```python
from build123d import *

# Parameters (mm, degrees)
SKETCH2_W           = 190.5
SKETCH2_H           = 203.2
BOSS_EXTRUDE1_DEPTH = 6
SKETCH5_R           = 2.5
CUT_EXTRUDE6_DEPTH  = 7
SKETCH6_W           = 31.9
SKETCH6_H           = 11
SKETCH6_R           = 2
CUT_EXTRUDE8_DEPTH  = 10


with BuildPart() as part:
    # Sketch2 → Boss-Extrude1 (new body)
    with BuildSketch(Plane(origin=(0, 0, 0), x_dir=(1, 0, 0), z_dir=(0, 1, 0))):
        Rectangle(SKETCH2_W, SKETCH2_H)
    extrude(amount=BOSS_EXTRUDE1_DEPTH)

    # Sketch5 → Cut-Extrude6 (cut, through all)
    with BuildSketch(Plane(origin=(0, 6, 0), x_dir=(1, 0, 0), z_dir=(0, 1, 0))):
        with Locations((-78.187036158, 94.165073798)):
            Circle(SKETCH5_R)
        with Locations((0, 94.165073798)):
            Circle(SKETCH5_R)
        with Locations((78.187036158, 0)):
            Circle(SKETCH5_R)
        with Locations((-78.187036158, 0)):
            Circle(SKETCH5_R)
        with Locations((78.187036158, 94.165073798)):
            Circle(SKETCH5_R)
        with Locations((-78.187036158, -94.165073798)):
            Circle(SKETCH5_R)
        with Locations((78.187036158, -94.165073798)):
            Circle(SKETCH5_R)
    extrude(amount=-CUT_EXTRUDE6_DEPTH, mode=Mode.SUBTRACT)

    # Sketch6 → Cut-Extrude8 (cut)
    with BuildSketch(Plane(origin=(0, 6, 0), x_dir=(1, 0, 0), z_dir=(0, 1, 0))):
        with Locations((-40, -79.526039011)):
            Rectangle(SKETCH6_W, SKETCH6_H)
        Polygon((-30, 28.326034404), (-15.95, 28.326034404), (20, 28.326034404), (30, 28.326034404), (30, 88.326034404), (-30, 88.326034404), align=None)
        with Locations((40, -79.526039011)):
            Rectangle(SKETCH6_W, SKETCH6_H)
        with Locations((15.95, -10.676039011)):
            Circle(SKETCH6_R)
        with Locations((-15.95, -10.676039011)):
            Circle(SKETCH6_R)
        with Locations((-15.95, -42.576039011)):
            Circle(SKETCH6_R)
        with Locations((15.95, -42.576039011)):
            Circle(SKETCH6_R)
    extrude(amount=-CUT_EXTRUDE8_DEPTH, mode=Mode.SUBTRACT)


solid = part.part
```
Source: CAD feature listing. Evaluate the final solid. Frame: model axes, mm. A direction names the side the tool comes from. Coordinates: 2 decimals unless noted, no trailing zeros. Order: outer loops, then holes, each group sorted by start corner. A loop starts at its lowest first (then second) coordinate and runs counter-clockwise, first axis right, second up. Notation, with made-up numbers: M 29,54.5 L 74,54.5 A16 cw 74,59.5 Z; hole C -35.5,39 d4. An arc over 180 degrees is marked long. Write each question's results on one line, items separated by ' | '. Start each with the question number.
1) Section query A-A (x = -32.5). Return the cut outline in (y, z).
2) Draft query along Z for faces 1 (the face through (-95.25, 3, 1)), 2 (the face through (-1, 3, -101.6)), 3 (the face through (0, 3, -28.326)). Return one class per face: released by +Z, released by -Z, zero draft, split by the parting line, or undercut.
3) Line query: line 1 (X direction, y = 2.85, z = 77); line 2 (Z direction, x = -27.5, y = 3.55); line 3 (Z direction, x = -15.95, y = 4.65). Output: solid intervals per line, ascending. Write a range as from..to.
4) Access query for faces 4 (the face through (-30, 3, -59)), 5 (the face through (-1, 3, 101.6)). Directions: +Z, -Z, +X, -X, +Y, -Y. A direction counts if a zero-diameter tool reaches every point of the face in a straight line with its end or side. Return the directions, or none.
5) Contact query for a flat-ended pin moving along its axis: pin 1 Ø3.5 at (x, z) = (15.95, 42.58) entering from -Y. Output: stop coordinate, or through.
6) Section query B-B (x = 0). Return the cut outline in (y, z).
7) Section query C-C (z = -47). Return the cut outline in (x, y).
8) Section query D-D (y = 3.85). Give the number of separate pieces and of enclosed holes in the cut face, plus the area to 3 significant figures.
Answers:
1) outline: M 0,-101.6 L 6,-101.6 L 6,74.03 L 0,74.03 Z; M 0,85.03 L 6,85.03 L 6,101.6 L 0,101.6 Z
2) face 1: zero draft | face 2: released by -Z | face 3: undercut
3) line 1: x = -95.25..-55.95, -24.05..24.05, 55.95..95.25 | line 2: z = -101.6..-88.33, -28.33..74.03, 85.03..101.6 | line 3: z = -101.6..-88.33, -28.33..8.68, 12.68..40.58, 44.58..101.6
4) face 4: +Y, -Y | face 5: +Z, +X, -X, +Y, -Y
5) pin 1: passes through
6) outline: M 0,-101.6 L 6,-101.6 L 6,-96.67 L 0,-96.67 Z; M 0,-91.67 L 6,-91.67 L 6,-88.33 L 0,-88.33 Z; M 0,-28.33 L 6,-28.33 L 6,101.6 L 0,101.6 Z
7) outline: M -95.25,0 L -30,0 L -30,6 L -95.25,6 Z; M 30,0 L 95.25,0 L 95.25,6 L 30,6 Z
8) separate pieces: 1 | enclosed holes: 14 | area: 34,200 mm^2
